Work out the finished part from the listing and answer in its coordinate system (mm). Coordinates: 2 decimals unless noted, no trailing zeros. Order: outer loops, then holes, each group sorted by start corner. A loop starts at its lowest first (then second) coordinate and runs counter-clockwise, first axis right, second up. Notation, with made-up numbers: M -25.5,27 L 5.5,27 A6 ccw 5.5,31 Z; hole C 67,-9 d7. An arc over 180 degrees is marked long. Use a Markdown table: item, result.
from build123d import *

# Parameters (mm, degrees)
CYLINDER013_R     = 2
CYLINDER013_DEPTH = 140
BOX018_W          = 146
BOX018_H          = 30
BOX018_DEPTH      = 3


with BuildPart() as cilindro012:
    # Cylinder013 → Cylinder013 (new body)
    with BuildSketch(Plane(origin=(5, 404.5, 97), x_dir=(0, 0, -1), z_dir=(1, 0, 0))):
        Circle(CYLINDER013_R)
    extrude(amount=CYLINDER013_DEPTH)


with BuildPart() as fusion014006:
    # Box018 → Box018 (new body)
    with BuildSketch(Plane(origin=(2, 390, 96.5), x_dir=(1, 0, 0), z_dir=(0, 0, 1))):
        with Locations((73, 15)):
            Rectangle(BOX018_W, BOX018_H)
    extrude(amount=BOX018_DEPTH)

    # Fusion014006: union Cilindro012
    add(cilindro012.part)


solid = fusion014006.part
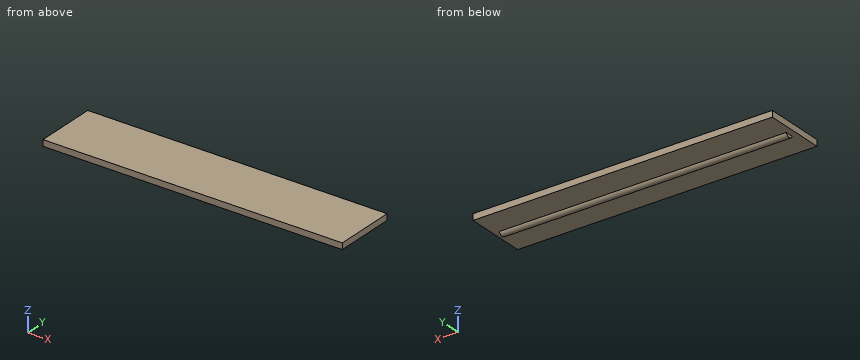
(1) Given P1, Ø12, axis at x = 73, y = 396.5, coming from the -Z side; P2, Ø0.8, axis at y = 405, z = 96, coming from the +X side, each flat-ended and moving along its own axis, determine where each tip first touches the part or whether it passes through.
Conclusion:
| item | result |
|---|---|
| P1 | z = 96.5 |
| P2 | x = 145 |
(2) Straight lines are drawn through the part: L1, parallel to Z at x = 138, y = 416.25; L2, parallel to Z at x = 10.5, y = 402.75; L3, parallel to Y at x = 42, z = 95.2. For each, find the intervals that lie inside material, in ascending order.
Conclusion:
| item | result |
|---|---|
| L1 | 96.5 to 99.5 |
| L2 | 96.03 to 99.5 |
| L3 | 403.63 to 405.37 |
(3) A cutting plane is placed at B-B (y = 410). Determine the outline of the cut face in (x, z), then the cut area to 3 significant figures.
Conclusion:
| item | result |
|---|---|
| outline | M 2,96.5 L 148,96.5 L 148,99.5 L 2,99.5 Z |
| area | 438 mm2 |
(4) A cutting plane is placed at A-A (x = 33). Determine the outline of the cut face in (y, z).
Conclusion:
| item | result |
|---|---|
| outline | M 390,96.5 L 402.56,96.5 A2 ccw 406.44,96.5 L 420,96.5 L 420,99.5 L 390,99.5 Z |
